```python
from build123d import *

# Parameters (mm, degrees)
SKETCH_1_R           = 3.5
EXTRUDE_1_DEPTH      = 27.5
SKETCH_2_R           = 2.25
CUT_EXTRUDE_1_DEPTH  = 8.2
SKETCH_3_W           = 40
SKETCH_3_H           = 7
EXTRUDE_2_DEPTH      = 1.25
SKETCH_3_4_R         = 1.6
CUT_EXTRUDE_3_DEPTH  = 1.5
EXTRUDE_3_DEPTH      = 0.5
EXTRUDE_3_DEPTH_BACK = 0.75


with BuildPart() as part:
    # Sketch 1 → Extrude 1 (new body)
    with BuildSketch(Plane.XY):
        Circle(SKETCH_1_R)
    extrude(amount=EXTRUDE_1_DEPTH)

    # Sketch 2 → Cut-Extrude 1 (cut)
    with BuildSketch(Plane(origin=(0, 0, 0), x_dir=(-1, 0, 0), z_dir=(0, 0, -1))):
        Circle(SKETCH_2_R)
    extrude(amount=-CUT_EXTRUDE_1_DEPTH, mode=Mode.SUBTRACT)

    # Sketch 3 → Extrude 2 (add)
    with BuildSketch(Plane.XY.offset(27.5)):
        Rectangle(SKETCH_3_W, SKETCH_3_H)
    extrude(amount=EXTRUDE_2_DEPTH)

    # Sketch 3_4 → Cut-Extrude 3 (cut)
    with BuildSketch(Plane.XY.offset(27.5)):
        with Locations((-16, 0)):
            Circle(SKETCH_3_4_R)
        with Locations((16, 0)):
            Circle(SKETCH_3_4_R)
    extrude(amount=CUT_EXTRUDE_3_DEPTH, mode=Mode.SUBTRACT)

    # Sketch 6 → Extrude 3 (add, two sides: drawn at the far end of the back side and taken through both)
    with BuildSketch(Plane(origin=(0, 3.5, 0), x_dir=(1, 0, 0), z_dir=(0, 1, 0)).offset(-EXTRUDE_3_DEPTH_BACK)):
        with BuildLine():
            ThreePointArc((0, -7.975), (-6.4, -14.375), (0, -20.775))
            Line((0, -20.775), (0, -7.975))
        make_face()
        with BuildLine():
            Line((0, -7.975), (0, -20.775))
            ThreePointArc((0, -20.775), (4.5254834, -18.9004834), (6.4, -14.375))
            ThreePointArc((6.4, -14.375), (4.5254834, -9.8495166), (0, -7.975))
        make_face()
        with BuildLine():
            ThreePointArc((0, -2.375), (-12, -14.375), (0, -26.375))
            Line((0, -26.375), (0, -23.975))
            ThreePointArc((0, -23.975), (-9.6, -14.375), (0, -4.775))
            Line((0, -4.775), (0, -2.375))
        make_face()
        with BuildLine():
            Line((0, -23.975), (0, -26.375))
            ThreePointArc((0, -26.375), (8.485281374, -22.860281374), (12, -14.375))
            ThreePointArc((12, -14.375), (8.485281374, -5.889718626), (0, -2.375))
            Line((0, -2.375), (0, -4.775))
            ThreePointArc((0, -4.775), (6.788225099, -7.586774901), (9.6, -14.375))
            ThreePointArc((9.6, -14.375), (6.788225099, -21.163225099), (0, -23.975))
        make_face()
    extrude(amount=EXTRUDE_3_DEPTH + EXTRUDE_3_DEPTH_BACK)


solid = part.part
```
Input: part model. Units: mm. Frame: model coordinates. A direction names the side the tool comes from. Coordinates: 2 decimals unless noted, no trailing zeros. Write each loop counter-clockwise with the first axis right and the second up, starting at its lowest first coordinate (ties: lowest second). Pieces come first, ordered by that corner, then holes.
1) Set-up query: faces 4 (the cylindrical face through (14.4, 0.07, 28.12)), 5 (the flat face through (0, 0, 8.2)), 6 (the flat face through (0, 3.5, 28)). Return all of +Z, -Z, +X, -X, +Y, -Y with unobstructed straight access to the full face (end or side cutting, diameter ignored); none if empty.
2) Material intervals for line 1 along X through (y, z) = (0, 27.9); line 2 along Y through (x, z) = (0, 5); line 3 along X through (y, z) = (3.25, 17.5), sorted ascending.
3) Pin query (flat end, axial travel): pin 1 Ø4.5 at (x, z) = (4, 15) entering from -Y; pin 2 Ø0.6 at (x, z) = (-6, 28) entering from +Y; pin 3 Ø1.5 at (y, z) = (-0.5, 3.5) entering from +X; pin 4 Ø2.5 at (x, y) = (-16, 0) entering from -Z. Return the tip coordinate at first contact, or that it passes through.
4) Section D-D on x = -8.5. Output: boundary loops of the cut face in (y, z).
5) Section C-C on z = 7. Output: boundary loops of the cut face in (x, y), and give its area (3 significant figures).
6) Section A-A on x = -16. Output: boundary loops of the cut face in (y, z), and give its area (3 significant figures).
7) Section B-B on y = 0. Output: boundary loops of the cut face in (x, z).
8) Mould query, pull axis Y, two halves, no side actions, for faces 1 (the flat face through (0, 0, 28.75)), 2 (the cylindrical face through (-0.759, -3.417, 13.558)), 3 (the flat face through (-5, 4, 6)). Classes: pulls with the +Y half, pulls with the -Y half, needs draft (parallel to the pull), parting line crosses it, or undercut.
Check result:
1. face 4: +Z, -Z
1. face 5: -Z
1. face 6: +Z, +X, -X, +Y
2. line 1: x = -20 to -17.6, -14.4 to 14.4, 17.6 to 20
2. line 2: y = -3.5 to -2.25, 2.25 to 3.5
2. line 3: x = -11.59 to -9.08, -5.59 to 5.59, 9.08 to 11.59
3. pin 1: stops at y = -3.03
3. pin 2: stops at y = 3.5
3. pin 3: stops at x = 3.5
3. pin 4: passes through
4. outline: (-3.5, 27.5) - (3.5, 27.5) - (3.5, 28.75) - (-3.5, 28.75) - close; (2.75, 5.9) - (4, 5.9) - (4, 9.91) - (2.75, 9.91) - close; (2.75, 18.84) - (4, 18.84) - (4, 22.85) - (2.75, 22.85) - close
5. outline: (-9.47, 2.75) - (-6.15, 2.75) - (-6.15, 4) - (-9.47, 4) - close; circle Ø7 at (0, 0); (6.15, 2.75) - (9.47, 2.75) - (9.47, 4) - (6.15, 4) - close; hole circle Ø4.5 at (0, 0)
5. area: 30.9 mm2
6. outline: (-3.5, 27.5) - (-1.6, 27.5) - (-1.6, 28.75) - (-3.5, 28.75) - close; (1.6, 27.5) - (3.5, 27.5) - (3.5, 28.75) - (1.6, 28.75) - close
6. area: 4.75 mm2
7. outline: (-20, 27.5) - (-17.6, 27.5) - (-17.6, 28.75) - (-20, 28.75) - close; (-14.4, 27.5) - (-3.5, 27.5) - (-3.5, 0) - (-2.25, 0) - (-2.25, 8.2) - (2.25, 8.2) - (2.25, 0) - (3.5, 0) - (3.5, 27.5) - (14.4, 27.5) - (14.4, 28.75) - (-14.4, 28.75) - close; (17.6, 27.5) - (20, 27.5) - (20, 28.75) - (17.6, 28.75) - close
8. face 1: needs draft
8. face 2: undercut
8. face 3: pulls with the +Y half
